Part model, mm, in its own coordinate system. A direction names the side the tool comes from. Coordinates: 2 decimals unless noted, no trailing zeros.
```python
from build123d import *

# Parameters (mm, degrees)
CROQUIS3_R                                           = 3.175
SALIENTE_EXTRUIR2_DEPTH                              = 10.922
REFRENTADO_PARA_TORNILLO_CON_CABEZA_HUEC_D           = 2.9718
REFRENTADO_PARA_TORNILLO_CON_CABEZA_HUEC_CBORE_D     = 4.699
REFRENTADO_PARA_TORNILLO_CON_CABEZA_HUEC_CBORE_DEPTH = 16.637


with BuildPart() as part:
    # Croquis3 → Saliente-Extruir2 (new, symmetric)
    with BuildSketch(Plane.XY):
        Circle(CROQUIS3_R)
    extrude(amount=SALIENTE_EXTRUIR2_DEPTH, both=True)

    # Refrentado para tornillo con cabeza hueca de 1/41 (through all)
    with Locations(Plane(origin=(0, 0, -10.922), x_dir=(-1, 0, 0), z_dir=(0, 0, -1))):
        with Locations((0, 0)):
            CounterBoreHole(REFRENTADO_PARA_TORNILLO_CON_CABEZA_HUEC_D / 2, REFRENTADO_PARA_TORNILLO_CON_CABEZA_HUEC_CBORE_D / 2, REFRENTADO_PARA_TORNILLO_CON_CABEZA_HUEC_CBORE_DEPTH)

    # Croquis7 → Cortar-Revolución1 (revolve, cut)
    with BuildSketch(Plane(origin=(0, 0, 0), x_dir=(1, 0, 0), z_dir=(0, 1, 0)), mode=Mode.PRIVATE) as cortar_revoluci_n1_sk:
        Polygon((-3.175, -8.3058), (-1.841979519, -10.922), (-3.175, -10.922), align=None)
    revolve(cortar_revoluci_n1_sk.sketch.rotate(Axis((0, 0, 10.922), (0, 0, -1)), 180), axis=Axis((0, 0, 10.922), (0, 0, -1)), mode=Mode.SUBTRACT)


solid = part.part
```
(1) Tool access for faces 3 (the face through (-0.69, -3.1, -1.17)), 4 (the face through (0, -2, 5.715)): list every direction of +Z, -Z, +X, -X, +Y, -Y with a clear straight run to the whole face (end or side of a thin tool).
(2) Pull direction Y, two halves, no side cores. Call faces 1 (the face through (0.31, 2.33, -2.72)), 2 (the face through (1.96, -0.62, 10.5)): +Y half, -Y half, draft (parallel to the pull), parting line (faces both ways), or undercut.
(3) Probe line 1 (Y direction, x = 0, z = -3) (1 decimal); line 2 (Y direction, x = 0.75, z = 5.25); line 3 (X direction, y = -1.5, z = -8). List the from-to ranges inside material, lowest first.
(4) Drop flat-ended pins along their axis: pin 1 (3.5 mm diameter, centred on x = 0, y = 0, fed in from +Z); pin 2 (1.5 mm diameter, centred on x = 1.5, z = -8, fed in from -Y); pin 3 (1 mm diameter, centred on y = -1.5, z = 4, fed in from +X); pin 4 (2.5 mm diameter, centred on x = -0.5, y = 0, fed in from -Z) (3 decimals). Give the stop position or say it passes through.
Here are the results:
1. face 3: +Z, -Z
1. face 4: -Z
2. face 1: undercut
2. face 2: parting line
3. line 1: y = -3.2 to -2.3, 2.3 to 3.2
3. line 2: y = -3.09 to -2.23, 2.23 to 3.09
3. line 3: x = -2.8 to -1.81, 1.81 to 2.8
4. pin 1: stops at z = 10.92
4. pin 2: stops at y = -3.09
4. pin 3: stops at x = 3.01
4. pin 4: stops at z = 5.715
